Check sheet for the modelled part. Datum: model origin and axes. Units: mm. Round coordinates to 2 decimals unless told otherwise and drop trailing zeros. Write each loop counter-clockwise with the first axis right and the second up, starting at its lowest first coordinate (ties: lowest second). Pieces come first, ordered by that corner, then holes. Notation, with made-up numbers: M 3.5,9.25 L 38.5,9.25 A36 cw 38.5,44.25 Z; hole C -1.5,77 d10. An arc over 180 degrees is marked long. Answer in a Markdown table with one row per item.
Autodesk Inventor part; units mm, degrees
ref_plane "YZ Plane" through (0, 0, 0) normal (1, 0, 0) x (0, 1, 0)
ref_plane "XZ Plane" through (0, 0, 0) normal (0, 1, 0) x (-1, 0, 0)
ref_plane "XY Plane" through (0, 0, 0) normal (0, 0, 1) x (1, 0, 0)
sketch "Sketch1" plane through (0, 0, 0) normal (0, 0, 1) x (1, 0, 0)
  circle A0 centre (0, 0) radius 14
  line L0 (0, 0) -> (-47, 0) construction
  circle A1 centre (-47, 0) radius 9
  line L1 (-47.9574, 8.9489) -> (-1.4894, 13.9206)
  line L2 (-47.9574, -8.9489) -> (-1.4894, -13.9206)
  dimension "d0" = 18
  dimension "d1" = 28
  dimension "d2" = 47
extrude "Extrusion1" add sketch "Sketch1" along normal mid plane 3.5
sketch "Sketch2" plane through (0, 0, 1.75) normal (0, 0, 1) x (1, 0, 0)
  arc A0 (-1.4894, -13.9206) -> (-1.4894, 13.9206) centre (0, 0) ccw
hole "Hole1" at (0, 0, 1.75) direction (0, 0, -1) diameter 15.84 end through all
sketch "Sketch3" plane through (0, 0, 1.75) normal (0, 0, 1) x (1, 0, 0)
  arc A0 (-47.9574, 8.9489) -> (-47.9574, -8.9489) centre (-47, 0) ccw
hole "Hole2" at (-47, 0, 1.75) direction (0, 0, -1) diameter 9 end through all
properties part number "312-01-02" material "Steel"
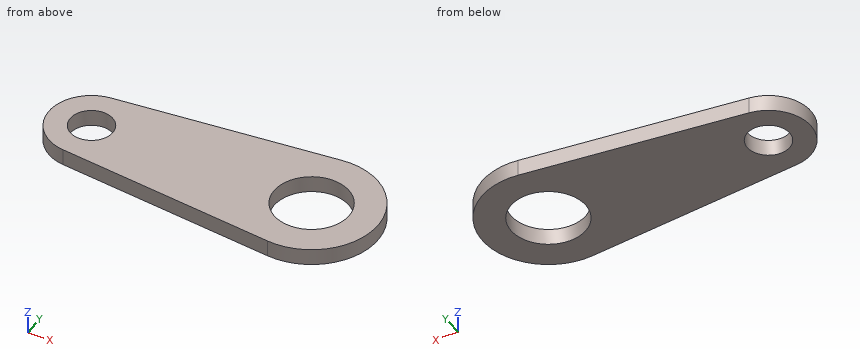
1. Go/stop test with a flat-tipped pin: pin 1 (1 mm diameter, centred on y = -8, z = -0.5, fed in from -X). Record where the tip stops, or that it passes through.
Found:
| item | result |
|---|---|
| pin 1 | stops at x = -51.97 |
2. Section check D-D, the plane z = 1. Record the cut outline in (x, y).
Found:
| item | result |
|---|---|
| outline | M -47.96,-8.95 L -1.49,-13.92 A14 ccw long -1.49,13.92 L -47.96,8.95 A9 ccw Z; hole C -47,0 d9; hole C 0,0 d15.84 |
3. Section check B-B, the plane y = 0. Record the cut outline in (x, z).
Found:
| item | result |
|---|---|
| outline | M -56,-1.75 L -51.5,-1.75 L -51.5,1.75 L -56,1.75 Z; M -42.5,-1.75 L -7.92,-1.75 L -7.92,1.75 L -42.5,1.75 Z; M 7.92,-1.75 L 14,-1.75 L 14,1.75 L 7.92,1.75 Z |
4. Section check A-A, the plane x = 0. Record the cut outline in (y, z).
Found:
| item | result |
|---|---|
| outline | M -14,-1.75 L -7.92,-1.75 L -7.92,1.75 L -14,1.75 Z; M 7.92,-1.75 L 14,-1.75 L 14,1.75 L 7.92,1.75 Z |
5. Section check C-C, the plane x = -47. Record the cut outline in (y, z), and give its area (3 significant figures).
Found:
| item | result |
|---|---|
| outline | M -9.05,-1.75 L -4.5,-1.75 L -4.5,1.75 L -9.05,1.75 Z; M 4.5,-1.75 L 9.05,-1.75 L 9.05,1.75 L 4.5,1.75 Z |
| area | 31.9 mm2 |
6. Scan lines: L1, parallel to Y at x = 0, z = -0.85; L2, parallel to X at y = 2.75, z = 0.3; L3, parallel to Y at x = -47, z = -0.2. Record each from-to range of solid material in increasing order.
Found:
| item | result |
|---|---|
| L1 | y = -14 to -7.92, 7.92 to 14 |
| L2 | x = -55.57 to -50.56, -43.44 to -7.43, 7.43 to 13.73 |
| L3 | y = -9.05 to -4.5, 4.5 to 9.05 |
